Design review of the part built by this model. Coordinates are the model's own, in mm. A direction names the side the tool comes from. Coordinates: 2 decimals unless noted, no trailing zeros. Loops run counter-clockwise (first coordinate to the right, second up) from the corner with the lowest first, then second, coordinate; pieces in that order, holes last. Notation, with made-up numbers: M 75.5,46 L 80.5,46 A31 cw 80.5,83 Z; hole C -36.5,-25 d5. An arc over 180 degrees is marked long. One line per item, written item: value.
Autodesk Inventor part; units mm, degrees
ref_plane "Work Plane1" through (0, 2.5, 0) normal (0, 1, 0) x (-1, 0, 0)
ref_plane "YZ Plane" through (0, 0, 0) normal (1, 0, 0) x (0, 1, 0)
ref_plane "XY Plane" through (0, 0, 0) normal (0, 0, 1) x (1, 0, 0)
sketch "Sketch1" plane through (0, 0, 0) normal (0, 0, 1) x (1, 0, 0)
  line L0 (0, 0) -> (0, 1.5)
  line L1 (0, 1.5) -> (4, 1.5)
  line L2 (4, 1.5) -> (4, 2.5)
  line L3 (4, 2.5) -> (16, 2.5)
  line L4 (16, 2.5) -> (16, 5)
  line L5 (16, 5) -> (18, 5)
  line L6 (18, 5) -> (18, 3)
  line L7 (18, 3) -> (23, 3)
  line L8 (23, 3) -> (23, 5)
  line L9 (23, 5) -> (28, 5)
  line L10 (28, 5) -> (28, 0)
  line L11 (28, 0) -> (0, 0)
  dimension "d0" = 28
  dimension "d1" = 5
  dimension "d2" = 5
  dimension "d3" = 2
  dimension "d4" = 12
  dimension "d5" = 3
  dimension "d6" = 5
  dimension "d7" = 10
  dimension "d8" = 6
revolve "Revolution1" add sketch "Sketch1" angle 360 about axis through (28, 0, 0) along (-1, 0, 0)
ref_plane "Work Plane1" through (0, 2.5, 0) normal (0, 1, 0) x (-1, 0, 0)
sketch "Sketch2" plane through (0, 2.5, 0) normal (0, 1, 0) x (-1, 0, 0)
  line L0 (-4, -2.5) -> (-4, 2.5)
  point P0 (0, 0)
  point P1 (-10, 0)
  dimension "d11" = 6
hole "Hole1" at (10, 2.5, 0) direction (0, -1, 0) diameter 3 end through all
thread "Thread1"
fillet "Fillet1" radius 0.5 2 edges at (18, -3, 0) (23, -3, 0)
sketch "Sketch4" plane through (0, 2.5, 0) normal (0, 1, 0) x (-1, 0, 0)
  line L0 (-28, -5) -> (-28, 5)
  point P0 (0, 0)
  point P1 (-25.5, 0)
  point P2 (-28, 0)
  dimension "d22" = 2.5
hole "Hole2" at (25.5, 2.5, 0) direction (0, 1, 0) diameter 3 end through all
thread "Thread2"
properties part number "141"
(1) We need section C-C on y = -4.5. State the section outline as (x, z) points.
Reply:
outline: M 16,-2.18 L 18,-2.18 L 18,2.18 L 16,2.18 Z; M 23,-2.18 L 28,-2.18 L 28,2.18 L 23,2.18 Z
(2) Mouldability with a two-part tool opening along X and no side actions: class faces 1 (the cylindrical face through (17.01, -1.08, -4.88)), 2 (the flat face through (4, 2, 0)), 3 (the flat face through (18, 2.2, 3.3)) as released by +X, released by -X, zero draft, split by the parting line, or undercut.
Reply:
face 1: zero draft
face 2: released by -X
face 3: undercut
(3) We need section D-D on x = 10. State the section outline as (y, z) points.
Reply:
outline: M -2,-1.5 A2.5 ccw 2,-1.5 Z; M -2,1.5 L 2,1.5 A2.5 ccw Z
(4) Tool access review of faces 4 (the flat face through (25, 2.5, 0)), 5 (the cylindrical face through (2.03, -1.5, 0.07)), 6 (the flat face through (23, 2.2, 3.3)): name each direction out of +Z, -Z, +X, -X, +Y, -Y from which nothing blocks a thin tool from reaching the whole face with its end or side.
Reply:
face 4: +Y
face 5: -X
face 6: none
(5) We need section B-B on y = 0. State the section outline as (x, z) points.
Reply:
outline: M 0,-1.5 L 4,-1.5 L 4,-2.5 L 16,-2.5 L 16,-5 L 18,-5 L 18,-3.5 A0.5 cw 18.5,-3 L 22.5,-3 A0.5 cw 23,-3.5 L 23,-5 L 28,-5 L 28,5 L 23,5 L 23,3.5 A0.5 cw 22.5,3 L 18.5,3 A0.5 cw 18,3.5 L 18,5 L 16,5 L 16,2.5 L 4,2.5 L 4,1.5 L 0,1.5 Z; hole C 10,0 d3
(6) To check wall thickness, follow line 1 along X through (y, z) = (3.8, 0); line 2 along X through (y, z) = (-2.75, 2.5); line 3 along X through (y, z) = (-0.8, 0). State the ranges of each line that lie inside material, in increasing order. Write a range as [from, to].
Reply:
line 1: x = [16, 18], [23, 24], [27, 28]
line 2: x = [16, 18], [23, 28]
line 3: x = [0, 8.5], [11.5, 28]
(7) Insertion check: pin 1 (2 mm diameter, centred on x = 18, y = 1.5, fed in from -Z); pin 2 (1.5 mm diameter, centred on x = 6.5, y = -1, fed in from -Z); pin 3 (5 mm diameter, centred on x = 10.5, z = 3, fed in from -Y); pin 4 (1.8 mm diameter, centred on x = 10, z = 0, fed in from +Y). Each pin has a flat end and moves straight along its axis. Give the tip position at first contact, or say it passes through.
Reply:
pin 1: stops at z = -4.97
pin 2: stops at z = -2.49
pin 3: stops at y = -2.41
pin 4: passes through
